Input: part model. Units: mm. Frame: model coordinates. Face numbers are marked on the shaded views. A direction names the side the tool comes from. Coordinates: 2 decimals unless noted, no trailing zeros. Loops run counter-clockwise (first coordinate to the right, second up) from the corner with the lowest first, then second, coordinate; pieces in that order, holes last.
Item 1: Section C-C on z = 34. Return loops of the section in (x, y), and give its area (3 significant figures).
Item 2: Section D-D on x = 16. Return loops of the section in (y, z).
Item 3: Ray query, line 1 along X through (y, z) = (-18, 15.5); line 2 along Z through (x, y) = (-1.5, -4.25); line 3 along X through (y, z) = (-19.5, 12). Return the intervals inside material, ascending.
Item 4: Pull-direction query (Z, two-part tool) for the marked faces 4, 5 and 6; classes: released by +Z, released by -Z, zero draft, split by the parting line, or undercut.
Item 5: Section A-A on y = -14. Return loops of the section in (x, z).
Item 6: Reachability of the marked faces 1, 2 and 3 from +Z, -Z, +X, -X, +Y, -Y: full face, straight path, thin tool, end or side. Return the list, or none.
Item 7: Section B-B on y = -2. Return loops of the section in (x, z), and give its area (3 significant figures).
Item 8: Contact query for flat-ended pins moving along their axis: P1, Ø4.5, axis at x = 11.83, z = 33.28, coming from the -Y side; P2, Ø2, axis at x = 14.5, z = -4.5, coming from the -Y side; P3, Ø6, axis at x = 1, y = -8.5, coming from the +Z side; P4, Ø5, axis at x = 5.5, z = -5, coming from the -Y side. Output: stop coordinate, or through.
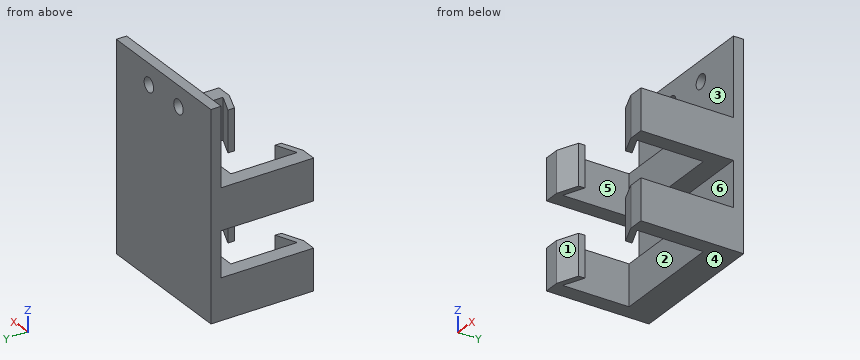
```python
from build123d import *

# Parameters (mm, degrees)
SKETCH3_W           = 35.56
SKETCH3_H           = 50.8
SKETCH3_R           = 1.778
BOSS_EXTRUDE3_DEPTH = 2.54
SKETCH4_W           = 3.81
SKETCH4_H           = 36.576
BOSS_EXTRUDE4_DEPTH = 22.86
SKETCH5_W           = 36.576
SKETCH5_H           = 1.524
BOSS_EXTRUDE5_DEPTH = 5.08
SKETCH6_W           = 36.576
SKETCH6_H           = 1.524
BOSS_EXTRUDE6_DEPTH = 5.08
SKETCH7_W           = 35.56
SKETCH7_H           = 22.86
CUT_EXTRUDE1_DEPTH  = 5.08
SKETCH11_W          = 35.56
SKETCH11_H          = 31.496
BOSS_EXTRUDE7_DEPTH = 4.9022
BOSS_EXTRUDE8_DEPTH = 31.496
SKETCH8_W           = 11.176
SKETCH8_H           = 22.86
CUT_EXTRUDE2_DEPTH  = 36.56
CUT_EXTRUDE3_DEPTH  = 32.496


with BuildPart() as part:
    # Sketch3 → Boss-Extrude3 (new body)
    with BuildSketch(Plane(origin=(0, 0, 0), x_dir=(1, 0, 0), z_dir=(0, 1, 0))):
        with Locations((6.262748092, -12.959016216)):
            Rectangle(SKETCH3_W, SKETCH3_H)
        with Locations((0.700148092, -33.279016216)):
            Circle(SKETCH3_R, mode=Mode.SUBTRACT)
        with Locations((11.825348092, -33.279016216)):
            Circle(SKETCH3_R, mode=Mode.SUBTRACT)
    extrude(amount=BOSS_EXTRUDE3_DEPTH)

    # Sketch4 → Boss-Extrude4 (add)
    with BuildSketch(Plane.XZ):
        with Locations((-9.612251908, 5.847016216)):
            Rectangle(SKETCH4_W, SKETCH4_H)
        with Locations((22.137748092, 5.847016216)):
            Rectangle(SKETCH4_W, SKETCH4_H)
    extrude(amount=BOSS_EXTRUDE4_DEPTH)

    # Sketch5 → Boss-Extrude5 (add)
    with BuildSketch(Plane(origin=(-7.707251908, 0, 0), x_dir=(0, 0, -1), z_dir=(1, 0, 0))):
        with Locations((-5.847016216, -22.098)):
            Rectangle(SKETCH5_W, SKETCH5_H)
    extrude(amount=BOSS_EXTRUDE5_DEPTH)

    # Sketch6 → Boss-Extrude6 (add)
    with BuildSketch(Plane.ZY.offset(-20.232748092)):
        with Locations((5.847016216, -22.098)):
            Rectangle(SKETCH6_W, SKETCH6_H)
    extrude(amount=BOSS_EXTRUDE6_DEPTH)

    # Sketch7 → Cut-Extrude1 (cut)
    with BuildSketch(Plane.XY.offset(24.135016216)):
        with Locations((6.262748092, -11.43)):
            Rectangle(SKETCH7_W, SKETCH7_H)
    extrude(amount=-CUT_EXTRUDE1_DEPTH, mode=Mode.SUBTRACT)

    # Sketch11 → Boss-Extrude7 (add)
    with BuildSketch(Plane.XZ):
        with Locations((6.262748092, 3.307016216)):
            Rectangle(SKETCH11_W, SKETCH11_H)
    extrude(amount=BOSS_EXTRUDE7_DEPTH)

    # Sketch12 → Boss-Extrude8 (add)
    with BuildSketch(Plane.XY.offset(19.055016216)):
        Polygon((-7.707251908, -21.336), (-2.593407451, -19.20881978), (-2.627251908, -21.336), align=None)
        Polygon((15.152748092, -21.336), (15.152748092, -19.20881978), (20.232748092, -21.336), align=None)
    extrude(amount=-BOSS_EXTRUDE8_DEPTH)

    # Sketch8 → Cut-Extrude2 (cut, through all)
    with BuildSketch(Plane(origin=(24.042748092, 0, 0), x_dir=(0, 0, -1), z_dir=(1, 0, 0))):
        with Locations((-3.307016216, -11.43)):
            Rectangle(SKETCH8_W, SKETCH8_H)
    extrude(amount=-CUT_EXTRUDE2_DEPTH, mode=Mode.SUBTRACT)

    # Sketch13 → Cut-Extrude3 (cut, through all)
    with BuildSketch(Plane.XY.offset(19.055016216)):
        Polygon((-7.660745747, -22.86), (-2.618035473, -20.756731792), (-2.627251908, -22.86), align=None)
        Polygon((15.152748092, -22.86), (20.204845905, -22.86), (15.152748092, -20.834602636), align=None)
    extrude(amount=-CUT_EXTRUDE3_DEPTH, mode=Mode.SUBTRACT)


solid = part.part
```
Results found:
1. outline: (-11.52, 0) - (-0.93, 0) - (-0.93, 2.54) - (-11.52, 2.54) - close; (2.33, 0) - (10.2, 0) - (10.2, 2.54) - (2.33, 2.54) - close; (13.45, 0) - (24.04, 0) - (24.04, 2.54) - (13.45, 2.54) - close
1. area: 73.8 mm2
2. outline: (-21.17, -12.44) - (-19.56, -12.44) - (-19.56, -2.28) - (-21.17, -2.28) - close; (-21.17, 8.9) - (-19.56, 8.9) - (-19.56, 19.06) - (-21.17, 19.06) - close; (-4.9, -12.44) - (2.54, -12.44) - (2.54, 38.36) - (0, 38.36) - (0, 19.06) - (-4.9, 19.06) - (-4.9, 8.9) - (0, 8.9) - (0, -2.28) - (-4.9, -2.28) - close
3. line 1: x = -11.52 to -7.71, 20.23 to 24.04
3. line 2: z = -12.44 to -2.28, 8.9 to 19.06
3. line 3: x = -11.52 to -7.71, -3.29 to -2.6, 15.15 to 15.85, 20.23 to 24.04
4. face 4: released by -Z
4. face 5: zero draft
4. face 6: undercut
5. outline: (-11.52, -12.44) - (-7.71, -12.44) - (-7.71, -2.28) - (-11.52, -2.28) - close; (-11.52, 8.9) - (-7.71, 8.9) - (-7.71, 19.06) - (-11.52, 19.06) - close; (20.23, -12.44) - (24.04, -12.44) - (24.04, -2.28) - (20.23, -2.28) - close; (20.23, 8.9) - (24.04, 8.9) - (24.04, 19.06) - (20.23, 19.06) - close
6. face 1: +Z, -Z, -Y
6. face 2: +Z, -Z
6. face 3: +Z, +X, -X, -Y
7. outline: (-11.52, -12.44) - (24.04, -12.44) - (24.04, -2.28) - (-11.52, -2.28) - close; (-11.52, 8.9) - (24.04, 8.9) - (24.04, 19.06) - (-11.52, 19.06) - close
7. area: 723 mm2
8. P1: stops at y = 0
8. P2: stops at y = -20.97
8. P3: passes through
8. P4: stops at y = -4.9
